from build123d import *

# Parameters (mm, degrees)
BOSS_EXTRU_1_DEPTH      = 15
ESQUISSE2_R             = 4
ENL_V_MAT_EXTRU_2_DEPTH = 60
ESQUISSE4_R             = 4
ENL_V_MAT_EXTRU_3_DEPTH = 60


with BuildPart() as part:
    # Esquisse1 → Boss.-Extru.1 (new body)
    with BuildSketch(Plane.XY):
        Polygon((60, -80.714285714), (123.820965425, -120.714285714), (-123.82, -120.714285714), (-60, -80.714285714), (-60, 79.285714286), (-90, 79.285714286), (0, 179.686053035), (90, 79.285714286), (60, 79.285714286), align=None)
    extrude(amount=BOSS_EXTRU_1_DEPTH)

    # Esquisse2 → Enlèv. mat.-Extru.2 (cut)
    with BuildSketch(Plane.XY.offset(15)):
        with Locations((0, 71.092567552)):
            Circle(ESQUISSE2_R)
    extrude(amount=-ENL_V_MAT_EXTRU_2_DEPTH, mode=Mode.SUBTRACT)

    # Esquisse4 → Enlèv. mat.-Extru.3 (cut)
    with BuildSketch(Plane.XY.offset(15)):
        with Locations((30, 11.786912572)):
            Circle(ESQUISSE4_R)
        with Locations((39.013840353, -50.053697219)):
            Circle(ESQUISSE4_R)
        with Locations((-30, 11.786912572)):
            Circle(ESQUISSE4_R)
        with Locations((-30, -50.053697219)):
            Circle(ESQUISSE4_R)
    extrude(amount=-ENL_V_MAT_EXTRU_3_DEPTH, mode=Mode.SUBTRACT)


solid = part.part
Work out the finished part from the listing and answer in its coordinate system (mm). A direction names the side the tool comes from. Round coordinates to 2 decimals unless told otherwise and drop trailing zeros. Loops run counter-clockwise (first coordinate to the right, second up) from the corner with the lowest first, then second, coordinate; pieces in that order, holes last. Notation, with made-up numbers: M 9.25,8 L 51.25,8 A28 cw 51.25,30 Z; hole C 10.25,88.5 d5. An arc over 180 degrees is marked long. One line per question, with ' | ' between items. Start each with the question number.
(1) Flat-ended cylindrical pins translate along their axes: pin 1 Ø5 at (y, z) = (-36.5, 1.5) entering from +X; pin 2 Ø8 at (x, z) = (77, 12.5) entering from +Y; pin 3 Ø4 at (y, z) = (143.5, 4.5) entering from -X. Find the tip coordinate at first contact, or state that the pin passes through.
(2) For a pull along Y with two mould halves and no side action, classify faces 1 (the face through (2, -2, 0)), 2 (the face through (35.84, -52.49, 7.6)), 3 (the face through (44.37, 130.19, 7.4)) as released by +Y, released by -Y, zero draft, split by the parting line, or undercut.
(3) A cutting plane is placed at D-D on y = 63. Write down the section's boundary in (x, z), plus the area to 3 significant figures.
(4) A tool of negligible diameter and unlimited length cuts with its end or side. For faces 4 (the face through (-75, 79.286, 7)), 5 (the face through (-30.867, 7.882, 7.605)), 6 (the face through (60, 0, 7)), from which of +Z, -Z, +X, -X, +Y, -Y can it reach the whole face along a straight path? Write none if from no direction.
(5) A cutting plane is placed at B-B on x = 30. Write down the section's boundary in (y, z).
(6) A cutting plane is placed at C-C on x = -30. Write down the section's boundary in (y, z).
(7) A cutting plane is placed at A-A on z = 3.75. Write down the section's boundary in (x, y).
(8) Find the intervals of material crossed by line 1 (X direction, y = 47, z = 5.5); line 2 (Y direction, x = -30, z = 6.25); line 3 (Y direction, x = -75, z = 1), in increasing order.
Geometry check:
1) pin 1: stops at x = 60 | pin 2: stops at y = 98.25 | pin 3: stops at x = -34.23
2) face 1: zero draft | face 2: undercut | face 3: released by +Y
3) outline: M -60,0 L 60,0 L 60,15 L -60,15 Z | area: 1,800 mm²
4) face 4: +Z, -Z, -X | face 5: +Z, -Z | face 6: +Z, -Z, +X
5) outline: M -120.71,0 L 7.79,0 L 7.79,15 L -120.71,15 Z; M 15.79,0 L 146.22,0 L 146.22,15 L 15.79,15 Z
6) outline: M -120.71,0 L -54.05,0 L -54.05,15 L -120.71,15 Z; M -46.05,0 L 7.79,0 L 7.79,15 L -46.05,15 Z; M 15.79,0 L 146.22,0 L 146.22,15 L 15.79,15 Z
7) outline: M -123.82,-120.71 L 123.82,-120.71 L 60,-80.71 L 60,79.29 L 90,79.29 L 0,179.69 L -90,79.29 L -60,79.29 L -60,-80.71 Z; hole C -30,-50.05 d8; hole C -30,11.79 d8; hole C 0,71.09 d8; hole C 30,11.79 d8; hole C 39.01,-50.05 d8
8) line 1: x = -60 to 60 | line 2: y = -120.71 to -54.05, -46.05 to 7.79, 15.79 to 146.22 | line 3: y = -120.71 to -90.12, 79.29 to 96.02
